Check sheet for the drawn part. Datum: minimum x, y, z corner. Units: mm. Round coordinates to 2 decimals unless told otherwise and drop trailing zeros. Order: outer loops, then holes, each group sorted by start corner. A loop starts at its lowest first (then second) coordinate and runs counter-clockwise, first axis right, second up. Notation, with made-up numbers: M -7,26 L 47,26 A26 ccw 47,41 Z; hole C -37.75,-19 d4. An arc over 180 degrees is marked long. Use one line per item in the form item = value. Start each with the question number.
Item 1: Release check for a two-part mould opening along X. For the marked faces 1 and 2 record: +X half, -X half, draft (parallel to the pull), parting line (faces both ways), or undercut.
Item 2: Go/stop test with flat-tipped pins: pin 1 Ø1.5 at (y, z) = (250.5, 29.5) entering from +X (1 decimal); pin 2 Ø1.5 at (y, z) = (119.5, 77.5) entering from +X; pin 3 Ø1.5 at (x, z) = (47, 39) entering from -Y. Record where each tip stops, or that it passes through.
Item 3: Cross-section at A-A on y = 152.4. Enter the section's corners in (x, z), then the cut area to 3 significant figures.
Item 4: Cross-section at C-C on z = 42. Enter the section's corners in (x, y).
Item 5: Cross-section at B-B on x = 70. Enter the section's corners in (y, z) (1 decimal).
Item 6: Thickness scan on probe 1 along Y at (x, z) = (152.4, 41); probe 2 along X at (y, z) = (172.5, 15.5). Record the ranges inside material, lowest first. Write a range as [from, to].
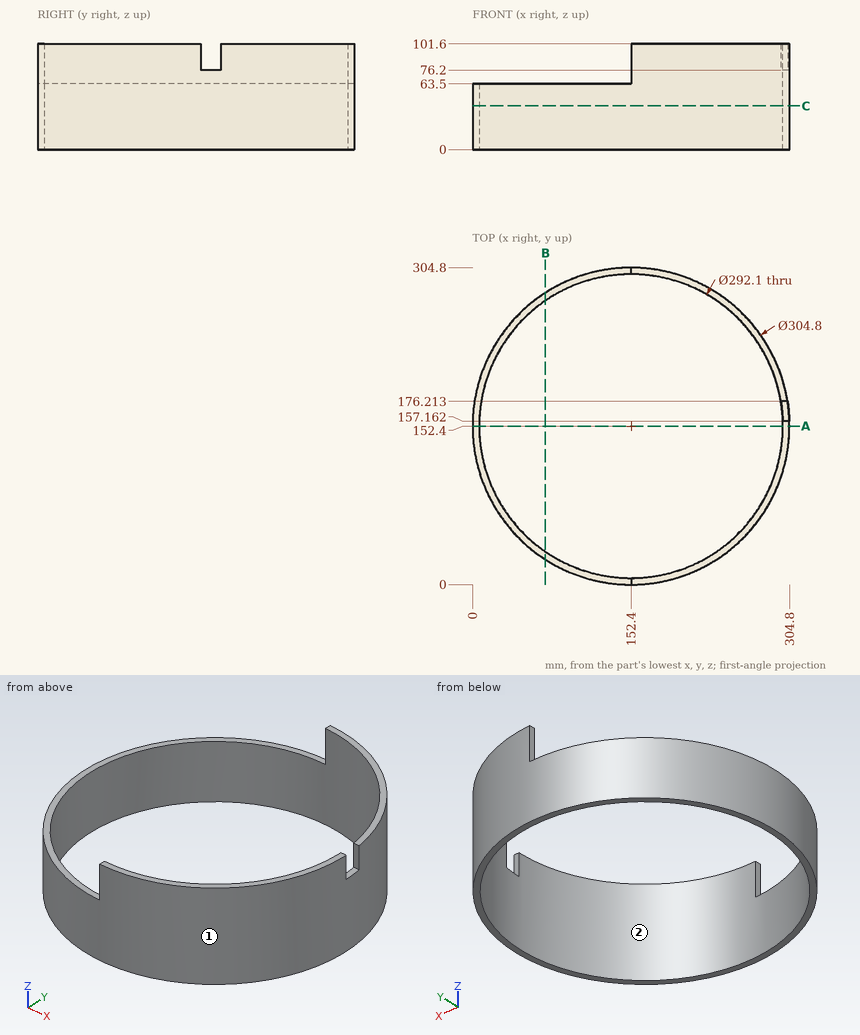
Output values:
q1.face_1 = parting line
q1.face_2 = undercut
q2.pin_1 = 269.7
q2.pin_2 = 301.37
q2.pin_3 = 41.61
q3.outline = M 0,0 L 6.35,0 L 6.35,63.5 L 0,63.5 Z; M 298.45,0 L 304.8,0 L 304.8,101.6 L 298.45,101.6 Z
q3.area = 1,050 mm2
q4.outline = C 152.4,152.4 d304.8; hole C 152.4,152.4 d292.1
q5.outline = M 24.2,0 L 31.8,0 L 31.8,63.5 L 24.2,63.5 Z; M 273,0 L 280.6,0 L 280.6,63.5 L 273,63.5 Z
q6.probe_1 = [0, 6.35], [298.45, 304.8]
q6.probe_2 = [1.33, 7.74], [297.06, 303.47]
